Geometry check sheet. Reference: drawing and pictorial views, mm from the part's lowest x, y, z. A direction names the side the tool comes from. Round coordinates to 2 decimals unless told otherwise and drop trailing zeros. Loops run counter-clockwise (first coordinate to the right, second up) from the corner with the lowest first, then second, coordinate; pieces in that order, holes last. Notation, with made-up numbers: (61, 40) - (72, 40) arc R27 cw to (72, 79) - close; hole circle Ø11 at (-36.5, 35). An arc over 180 degrees is marked (long way). Put each result on its own line as item: value. Start each with the question number.
Item 1: Gauge pin test, flat ends, axial feed: pin 1 Ø1.1 at (x, z) = (31.5, 20) entering from +Y; pin 2 Ø10 at (y, z) = (19, 32) entering from +X; pin 3 Ø1 at (x, y) = (43, 16.5) entering from +Z; pin 4 Ø10 at (x, y) = (20.5, 26.5) entering from +Z. Record the tip position at first contact, or that the pin passes through.
Item 2: Section check C-C, the plane x = 46.5. Record the cut outline in (y, z).
Item 3: Material ranges on line 1 along X through (y, z) = (30, 24); line 2 along Z through (x, y) = (27, 22); line 3 along Y through (x, z) = (8.5, 28), recorded low to high.
Item 4: Section check A-A, the plane y = 27.5. Record the cut outline in (x, z).
Item 5: Tool access check on the marked faces 4 and 5. Record the directions out of +Z, -Z, +X, -X, +Y, -Y that give a thin tool (end or side, any length) a straight path to the whole face; none if there is none.
Item 6: Section check D-D, the plane x = 18. Record the cut outline in (y, z), and give its area (3 significant figures).
Item 7: Section check B-B, the plane z = 26. Record the cut outline in (x, y).
Item 8: Draft check along X on the marked faces 1, 2 and 3. Enter one of: pulls with the +X half, pulls with the -X half, needs draft (parallel to the pull), parting line crosses it, or undercut.
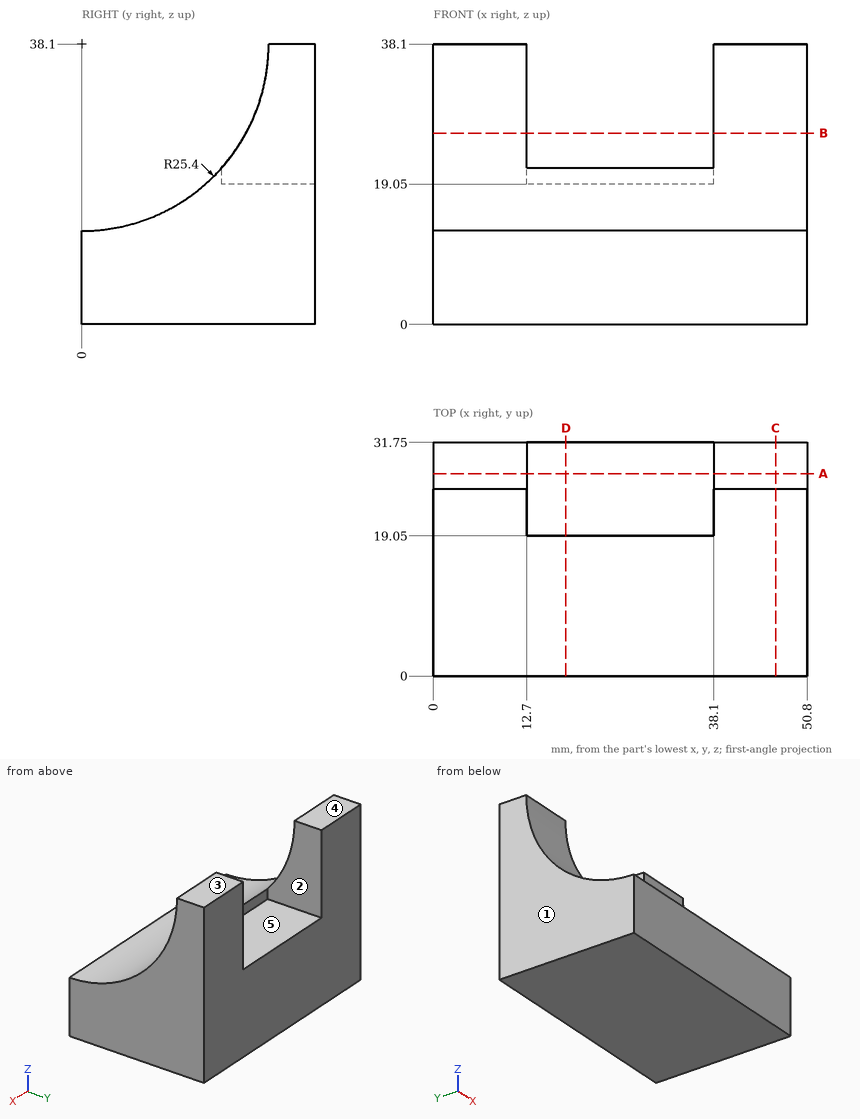
Check result:
1. pin 1: y = 19.05
1. pin 2: through
1. pin 3: z = 19.23
1. pin 4: z = 19.05
2. outline: (0, 0) - (31.75, 0) - (31.75, 38.1) - (25.4, 38.1) arc R25.4 cw to (0, 12.7) - close
3. line 1: 0 to 12.7, 38.1 to 50.8
3. line 2: 0 to 19.05
3. line 3: 23.31 to 31.75
4. outline: (0, 0) - (50.8, 0) - (50.8, 38.1) - (38.1, 38.1) - (38.1, 19.05) - (12.7, 19.05) - (12.7, 38.1) - (0, 38.1) - close
5. face 4: +Z, +X, -X, +Y, -Y
5. face 5: +Z, +Y
6. outline: (0, 0) - (31.75, 0) - (31.75, 19.05) - (19.05, 19.05) - (19.05, 21.3) arc R25.4 cw to (0, 12.7) - close
6. area: 534 mm²
7. outline: (0, 22.33) - (12.7, 22.33) - (12.7, 31.75) - (0, 31.75) - close; (38.1, 22.33) - (50.8, 22.33) - (50.8, 31.75) - (38.1, 31.75) - close
8. face 1: pulls with the -X half
8. face 2: undercut
8. face 3: needs draft
